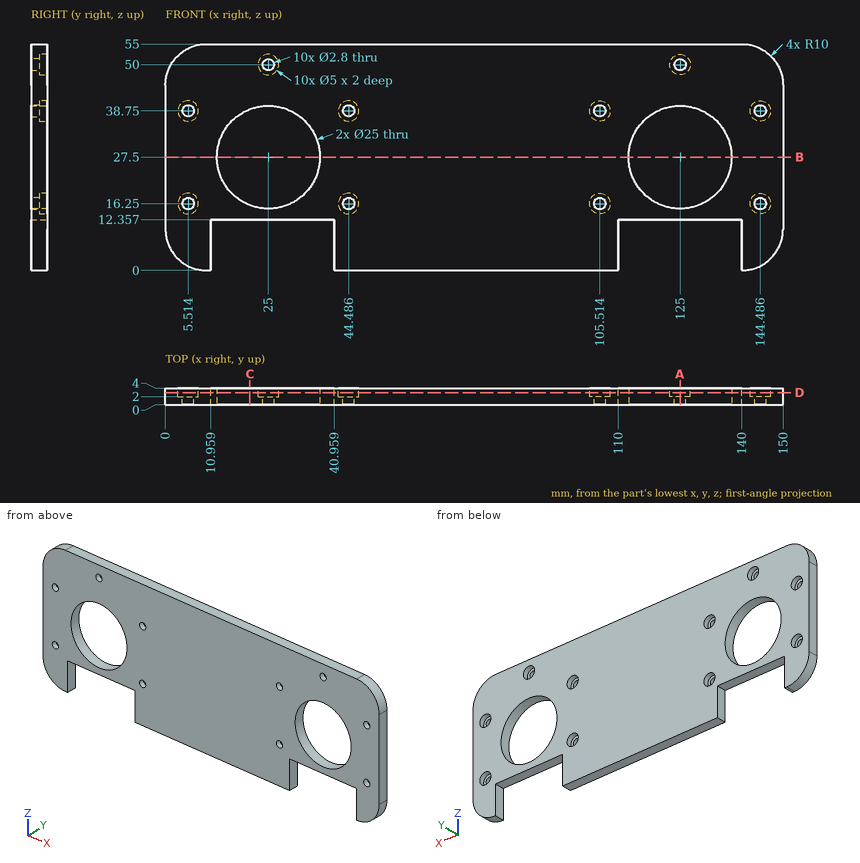
Here's the drawing with two shaded views (mm, measured from the low corner). I have some questions. Give positions to 0.01 mm unless a question says otherwise; leave off trailing zeros. Order: outer loops, then holes, each group sorted by start corner. A loop starts at its lowest first (then second) coordinate and runs counter-clockwise, first axis right, second up. Notation, with made-up numbers: (4.25, 86) -> (43.25, 86) arc R22 cw to (43.25, 119) -> close; hole circle Ø6 at (16.25, 69.5). An arc over 180 degrees is marked (long way). One line per item, written item: value. Start each with the question number.
1. Imagine slicing it at D-D, the plane y = 2.95. Count the separate pieces of the cut face and the enclosed holes in it.
2. Imagine slicing it at C-C, the plane x = 20.5. List the corners of the cut face in (y, z) for me.
3. Will these pins go through, and if not, where does the flat tip stop? pin 1 Ø3.5 at (x, z) = (44.49, 16.25) entering from -Y; pin 2 Ø2.5 at (x, z) = (44.5, 38) entering from +Y.
4. Imagine slicing it at B-B, the plane z = 27.5. List the corners of the cut face in (x, y) for me.
5. I need wall thicknesses on probe 1 along X at (y, z) = (0.45, 11.5); probe 2 along Z at (x, y) = (26, 3.7); probe 3 along X at (y, z) = (0.65, 34). Which ranges of each line are inside material? Lowest first, please. Write a range as from..to.
6. Imagine slicing it at A-A, the plane x = 125. List the corners of the cut face in (y, z) for me.
Values follow:
1. separate pieces: 1
1. enclosed holes: 12
2. outline: (0, 12.36) -> (4, 12.36) -> (4, 15.84) -> (0, 15.84) -> close; (0, 39.16) -> (4, 39.16) -> (4, 55) -> (0, 55) -> close
3. pin 1: stops at y = 0
3. pin 2: stops at y = 2
4. outline: (0, 0) -> (12.5, 0) -> (12.5, 4) -> (0, 4) -> close; (37.5, 0) -> (112.5, 0) -> (112.5, 4) -> (37.5, 4) -> close; (137.5, 0) -> (150, 0) -> (150, 4) -> (137.5, 4) -> close
5. probe 1: x = 0..10.96, 40.96..110, 140..150
5. probe 2: z = 12.36..15.04, 39.96..47.71, 52.29..55
5. probe 3: x = 0..14.32, 35.68..114.32, 135.68..150
6. outline: (0, 12.36) -> (4, 12.36) -> (4, 15) -> (0, 15) -> close; (0, 40) -> (4, 40) -> (4, 47.5) -> (2, 47.5) -> (2, 48.6) -> (0, 48.6) -> close; (0, 51.4) -> (2, 51.4) -> (2, 52.5) -> (4, 52.5) -> (4, 55) -> (0, 55) -> close
